Verification items for the finished model (mm, model axes). A direction names the side the tool comes from. Round coordinates to 2 decimals unless told otherwise and drop trailing zeros. Write each loop counter-clockwise with the first axis right and the second up, starting at its lowest first coordinate (ties: lowest second). Pieces come first, ordered by that corner, then holes. Notation, with made-up numbers: M 11.5,26.5 L 42.5,26.5 A15 cw 42.5,52.5 Z; hole C -18.5,47.25 d5. An arc over 180 degrees is marked long. Answer in a Markdown table with one row per item. Add a question column.
1. Draft check along X on faces 1 (the cylindrical face through (0.1, 12, -3.5)), 2 (the cylindrical face through (6.715, 7.178, -2.699)), 3 (the flat face through (0, 9, 4)), 4 (the flat face through (-8, 5, 0)). Enter one of: pulls with the +X half, pulls with the -X half, needs draft (parallel to the pull), parting line crosses it, or undercut.
2. Set-up check for faces 5 (the flat face through (-7, 7, 0)), 6 (the flat face through (0, 9, -4)): record each of +Z, -Z, +X, -X, +Y, -Y from which the full face is reachable in a straight line by a thin tool's end or side.
3. Sectioned sample at B-B on z = 0. Record the cut outline in (x, y), plus the area to 3 significant figures.
4. Material ranges on probe 1 along Z at (x, y) = (5.75, 6.5); probe 2 along X at (y, z) = (7, -0.25); probe 3 along Y at (x, z) = (-7, 3), recorded low to high.
5. Sectioned sample at C-C on x = 0. Record the cut outline in (y, z).
6. Sectioned sample at D-D on y = 6.25. Record the cut outline in (x, z), plus the area to 3 significant figures.
7. Sectioned sample at A-A on y = 8.5. Record the cut outline in (x, z), plus the area to 3 significant figures.
```python
from build123d import *

# Parameters (mm, degrees)
F1_DEPTH      = 4
F1_DEPTH_BACK = 4
F2_W          = 14
F2_H          = 6
F3_DEPTH      = 25
F4_R          = 1


with BuildPart() as f1:
    # F0 (on Top) → F1 (new body, two sides)
    with BuildSketch(Plane.XY) as f1_sk:
        with BuildLine():
            Line((8, 0), (8, 8.944272))
            ThreePointArc((8, 8.944272), (0, 12), (-8, 8.944272))
            Line((-8, 8.944272), (-8, 0))
            ThreePointArc((-8, 0), (0, 8), (8, 0))
        make_face()
    extrude(amount=F1_DEPTH)
    extrude(f1_sk.sketch, amount=-F1_DEPTH_BACK)

    # F2 (on Front) → F3 (cut)
    with BuildSketch(Plane.XZ):
        Rectangle(F2_W, F2_H)
    extrude(amount=-F3_DEPTH, mode=Mode.SUBTRACT)

    # F4
    f4_edges = [f1.edges().sort_by_distance(p)[0] for p in [
        (-7, 6.809889, 3),
        (-7, 6.809889, -3),
        (7, 6.809889, -3),
        (7, 6.809889, 3),
    ]]
    fillet(f4_edges, radius=F4_R)


solid = f1.part
```
Geometry check:
| question | item | result |
|---|---|---|
| 1 | face 1 | parting line crosses it |
| 1 | face 2 | undercut |
| 1 | face 3 | needs draft |
| 1 | face 4 | pulls with the -X half |
| 2 | face 5 | +Y, -Y |
| 2 | face 6 | -Z, +X, -X, +Y, -Y |
| 3 | outline | M -8,0 A8 cw -7,3.87 L -7,9.75 A12 ccw -8,8.94 Z; M 7,3.87 A8 cw 8,0 L 8,8.94 A12 ccw 7,9.75 Z |
| 3 | area | 13.5 mm2 |
| 4 | probe 1 | z = -4 to -3, 3 to 4 |
| 4 | probe 2 | x = -8 to -7, 7 to 8 |
| 4 | probe 3 | y = 3.87 to 9.75 |
| 5 | outline | M 8,-4 L 12,-4 L 12,-3 L 8,-3 Z; M 8,3 L 12,3 L 12,4 L 8,4 Z |
| 6 | outline | M -8,-4 L -4.99,-4 L -4.99,-3 L -6,-3 A1 cw -7,-2 L -7,2 A1 cw -6,3 L -4.99,3 L -4.99,4 L -8,4 Z; M 4.99,-4 L 8,-4 L 8,4 L 4.99,4 L 4.99,3 L 6,3 A1 cw 7,2 L 7,-2 A1 cw 6,-3 L 4.99,-3 Z |
| 6 | area | 24.9 mm2 |
| 7 | outline | M -8,-4 L 8,-4 L 8,4 L -8,4 Z; hole M -7,-2 A1 ccw -6,-3 L 6,-3 A1 ccw 7,-2 L 7,2 A1 ccw 6,3 L -6,3 A1 ccw -7,2 Z |
| 7 | area | 44.9 mm2 |
